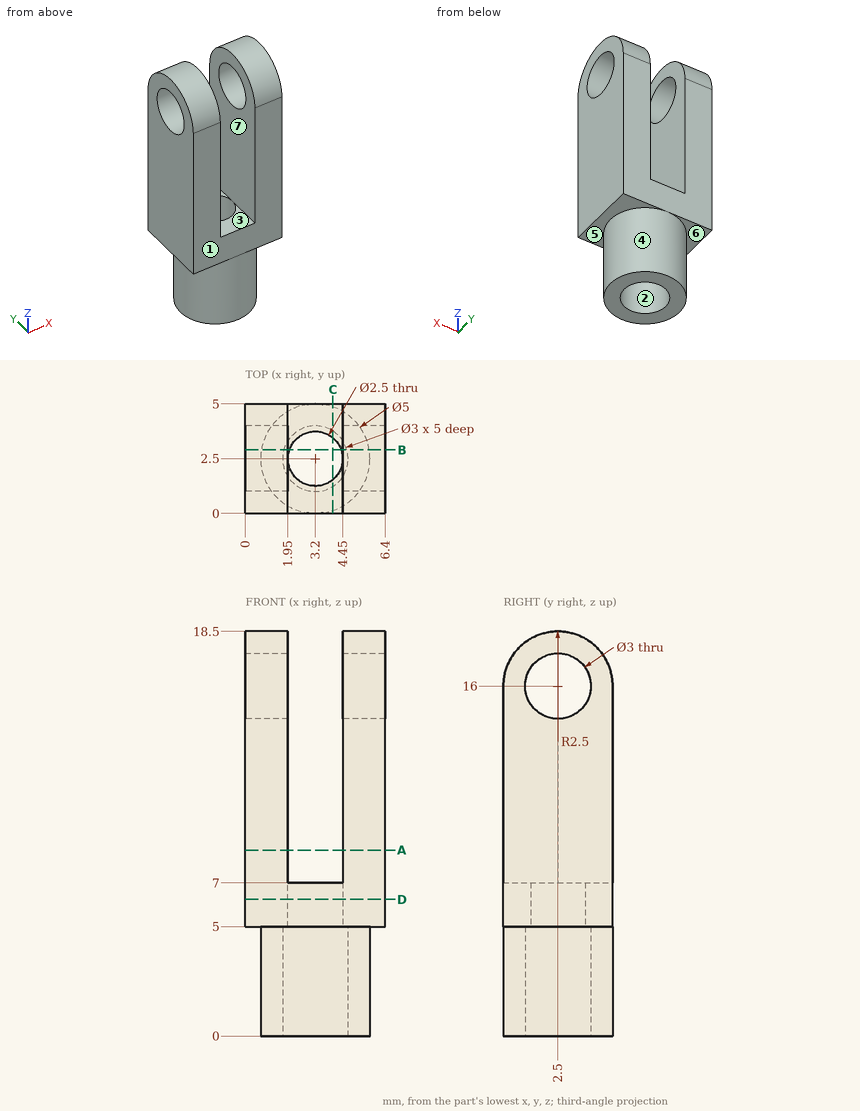
Can you work these out from the drawing? Everything is in mm from the part's minimum corner. A direction names the side the tool comes from. Give positions to 0.01 mm unless a question says otherwise; leave off trailing zeros. Loops run counter-clockwise (first coordinate to the right, second up) from the corner with the lowest first, then second, coordinate; pieces in that order, holes last. Notation, with made-up numbers: M 10.5,50 L 29.5,50 A11 cw 29.5,55 Z; hole C 3.25,-34 d6. An arc over 180 degrees is marked long. Use CSV: the item, a comma, the result in double quotes. Start each with the question number.
1. On a 3-axis mill with a long thin cutter (end or side, diameter ignored), from which of +Z, -Z, +X, -X, +Y, -Y can I reach the whole of each face in a straight line? I mean the marked faces 4, 5, 6 and 7. Say none if no direction works.
2. If I drill on L1, parallel to X at y = 4.65, z = 16.75; L2, parallel to Y at x = 3.2, z = 1.8; L3, parallel to Z at x = 5.6, y = 2.5, over which ranges is the centre line in solid material (lowest first)?
3. Imagine slicing it at B-B, the plane y = 2.9. Write out the boundary of the cut face in (x, z), plus the area to 3 significant figures.
4. Imagine slicing it at D-D, the plane z = 6.25. Write out the boundary of the cut face in (x, y), plus the area to 3 significant figures.
5. Imagine slicing it at C-C, the plane x = 4. Write out the boundary of the cut face in (y, z).
6. For P1, Ø1.5, axis at x = 3.2, y = 2.5, coming from the -Z side; P2, Ø0.8, axis at x = 3.5, y = 1.5, coming from the +Z side, each with a flat end and sliding along its axis, tell me the tip position at first contact or that it passes through.
7. Imagine slicing it at A-A, the plane z = 8.5. Write out the boundary of the cut face in (x, y), plus the area to 3 significant figures.
8. If we mould it in two halves opening along Y, with no side actions, what happens to the marked faces 1, 2 and 3? For each: released by +Y, released by -Y, zero draft, split by the parting line, or undercut.
Response values:
1,face 4,"-Z"
1,face 5,"-Z, +X"
1,face 6,"-Z, -X"
1,face 7,"+Z, +Y, -Y"
2,L1,"0 to 1.95, 4.45 to 6.4"
2,L2,"0 to 1, 4 to 5"
2,L3,"0 to 14.5, 17.5 to 18.5"
3,outline,"M 0,5 L 0.73,5 L 0.73,0 L 1.75,0 L 1.75,5 L 2.02,5 L 2.02,7 L 1.95,7 L 1.95,14.55 L 0,14.55 Z; M 0,17.45 L 1.95,17.45 L 1.95,18.47 L 0,18.47 Z; M 4.38,5 L 4.65,5 L 4.65,0 L 5.67,0 L 5.67,5 L 6.4,5 L 6.4,14.55 L 4.45,14.55 L 4.45,7 L 4.38,7 Z; M 4.45,17.45 L 6.4,17.45 L 6.4,18.47 L 4.45,18.47 Z"
3,area,"51.7 mm^2"
4,outline,"M 0,0 L 6.4,0 L 6.4,5 L 0,5 Z; hole C 3.2,2.5 d2.5"
4,area,"27.1 mm^2"
5,outline,"M 0,5 L 0.13,5 L 0.13,0 L 1.23,0 L 1.23,5 L 1.54,5 L 1.54,7 L 0,7 Z; M 3.46,5 L 3.77,5 L 3.77,0 L 4.87,0 L 4.87,5 L 5,5 L 5,7 L 3.46,7 Z"
6,P1,"through"
6,P2,"z = 7"
7,outline,"M 0,0 L 1.95,0 L 1.95,5 L 0,5 Z; M 4.45,0 L 6.4,0 L 6.4,5 L 4.45,5 Z"
7,area,"19.5 mm^2"
8,face 1,"released by -Y"
8,face 2,"undercut"
8,face 3,"zero draft"
